Autodesk Inventor part; units mm, degrees
ref_plane "YZ Plane" through (0, 0, 0) normal (1, 0, 0) x (0, 1, 0)
ref_plane "XZ Plane" through (0, 0, 0) normal (0, 1, 0) x (-1, 0, 0)
ref_plane "XY Plane" through (0, 0, 0) normal (0, 0, 1) x (1, 0, 0)
sketch "Sketch1" plane through (0, 0, 0) normal (0, 0, 1) x (1, 0, 0)
  line L0 (0, 0) -> (35.08, 0)
  line L1 (35.08, 0) -> (35.08, -60)
  line L2 (35.08, -60) -> (0, -60)
  line L3 (0, -60) -> (0, 0)
  dimension "d0" = 35.08
  dimension "d1" = 60
extrude "Extrusion1" add sketch "Sketch1" along normal blind 11
sketch "Sketch2" plane through (0, 0, 11) normal (0, 0, 1) x (1, 0, 0)
  line L0 (2, -3) -> (33.08, -3)
  line L1 (33.08, -3) -> (33.08, -57)
  line L2 (33.08, -57) -> (2, -57)
  line L3 (2, -57) -> (2, -3)
  line L4 (0, 0) -> (35.08, 0)
  line L5 (0, -60) -> (35.08, -60)
  line L6 (35.08, 0) -> (35.08, -60)
  line L7 (0, 0) -> (0, -60)
  dimension "d8" = 3
  dimension "d9" = 3
  dimension "d10" = 2
  dimension "d11" = 2
extrude "Extrusion2" cut sketch "Sketch2" against normal blind 9 contours L0 L1 L2 L3
sketch "Sketch4" plane through (0, -60, 0) normal (0, -1, 0) x (1, 0, 0)
  line L0 (2, 11) -> (2, 2)
  line L1 (2, 11) -> (2, 2)
  line L2 (2, 2) -> (4.5, 2)
  line L3 (2, 2) -> (33.08, 2)
  line L4 (4.5, 2) -> (4.5, 11)
  line L5 (2, 11) -> (4.5, 11)
  line L6 (0, 0) -> (0, 11)
  dimension "d22" = 9
  dimension "d23" = 4.5
extrude "Extrusion3" cut sketch "Sketch4" against normal blind 3
properties part number "prueba1Bateria"
Read the model definition and answer for the solid it produces. Units are mm, in the model's axes. A direction names the side the tool comes from. Round coordinates to 2 decimals unless told otherwise and drop trailing zeros. Write each loop counter-clockwise with the first axis right and the second up, starting at its lowest first coordinate (ties: lowest second). Pieces come first, ordered by that corner, then holes. Notation, with made-up numbers: (-23.5, -28) - (15.5, -28) arc R23 ccw to (15.5, 5) - close; hole circle Ø1 at (50.5, 89). An arc over 180 degrees is marked (long way). One line per item, written item: value.
Q1. For a pull along X with two mould halves and no side action, classify faces 4 (the flat face through (0, -30, 5)), 5 (the flat face through (35.08, -30, 5)), 6 (the flat face through (17, -3, 7)), 7 (the flat face through (18, -60, 5)) as pulls with the +X half, pulls with the -X half, needs draft (parallel to the pull), parting line crosses it, or undercut.
The answers:
face 4: pulls with the -X half
face 5: pulls with the +X half
face 6: undercut
face 7: needs draft
Q2. Find section A-A (x = 31). Determine the outline of the cut face in (y, z), and give its area (3 significant figures).
The answers:
outline: (-60, 0) - (0, 0) - (0, 11) - (-3, 11) - (-3, 2) - (-57, 2) - (-57, 11) - (-60, 11) - close
area: 174 mm2
Q3. This flat-tipped pin is pushed along its axis until it touches: P1, Ø9.5, axis at x = 17, y = -29, coming from the +Z side. Where does it stop, or does it pass through?
The answers:
P1: stops at z = 2
Q4. Find section B-B (z = 3.75). Determine the outline of the cut face in (x, y), and give its area (3 significant figures).
The answers:
outline: (0, -60) - (2, -60) - (2, -3) - (33.08, -3) - (33.08, -57) - (4.5, -57) - (4.5, -60) - (35.08, -60) - (35.08, 0) - (0, 0) - close
area: 419 mm2
Q5. Find section D-D (x = 3). Determine the outline of the cut face in (y, z), and give its area (3 significant figures).
The answers:
outline: (-60, 0) - (0, 0) - (0, 11) - (-3, 11) - (-3, 2) - (-60, 2) - close
area: 147 mm2
Q6. Find section C-C (y = -13.5). Determine the outline of the cut face in (x, z).
The answers:
outline: (0, 0) - (35.08, 0) - (35.08, 11) - (33.08, 11) - (33.08, 2) - (2, 2) - (2, 11) - (0, 11) - close
Q7. Which of the six approach directions +Z, -Z, +X, -X, +Y, -Y give full straight-line access (tool end or side, diameter ignored) to faces 1 (the flat face through (17, -30, 0)), 2 (the flat face through (19, -57, 7)), 3 (the flat face through (4.5, -59, 6))?
The answers:
face 1: -Z, +X, -X, +Y, -Y
face 2: +Z
face 3: +Z, -Y
Q8. Straight lines are drawn through the part: line 1 (X direction, y = -5.5, z = 4.5); line 2 (Y direction, x = 20.5, z = 5.5); line 3 (Z direction, x = 8, y = -47). For each, find the intervals that lie inside material, in ascending order. Write a range as from..to.
The answers:
line 1: x = 0..2, 33.08..35.08
line 2: y = -60..-57, -3..0
line 3: z = 0..2
